Here's the drawing with two shaded views (mm, measured from the low corner). I have some questions. Give positions to 0.01 mm unless a question says otherwise; leave off trailing zeros. Write each loop counter-clockwise with the first axis right and the second up, starting at its lowest first coordinate (ties: lowest second). Pieces come first, ordered by that corner, then holes. Notation, with made-up numbers: (-39, 62) -> (-32, 62) arc R21 cw to (-32, 99) -> close; hole circle Ø9 at (54.25, 14). An arc over 180 degrees is marked (long way). One line per question, with ' | ' between items.
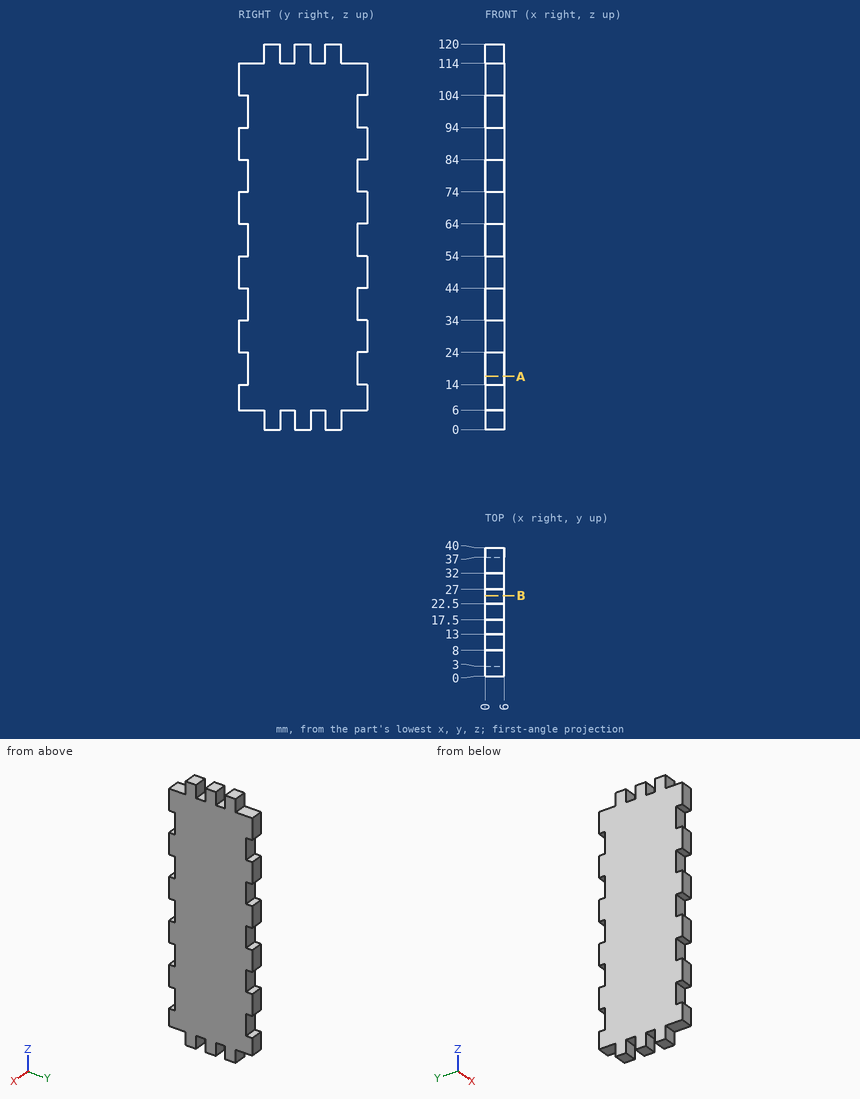
Q1. Imagine slicing it at B-B on y = 25. Please give me the cut outline in (x, z), and give its area (3 significant figures).
Answer below:
outline: (0, 6) -> (6, 6) -> (6, 114) -> (0, 114) -> close | area: 648 mm^2
Q2. If I drill on line 1 along Y through (x, z) = (4.45, 59); line 2 along Z through (x, y) = (4.4, 7.5), over which ranges is the centre line in solid material (lowest first)?
Answer below:
line 1: y = 3 to 37 | line 2: z = 6 to 114
Q3. Imagine slicing it at A-A on z = 16.5. Please give me the cut outline in (x, y).
Answer below:
outline: (0, 3) -> (6, 3) -> (6, 37) -> (0, 37) -> close
Q4. Will these pins go through, and if not, where does the flat tip stop? pin 1 (3 mm diameter, centred on x = 3.5, z = 19.5, fed in from -Y); pin 2 (1.3 mm diameter, centred on x = 4.5, y = 15, fed in from +Z); pin 3 (1 mm diameter, centred on x = 4.5, z = 36.5, fed in from +Y).
Answer below:
pin 1: stops at y = 3 | pin 2: stops at z = 114 | pin 3: stops at y = 37
